```python
from build123d import *

# Parameters (mm, degrees)
SKETCH1_R           = 1.1303
SKETCH1_R_2         = 0.889
SKETCH1_W           = 5
SKETCH1_H           = 8.000000002
BOSS_EXTRUDE1_DEPTH = 6.35


with BuildPart() as part:
    # Sketch1 → Boss-Extrude1 (new body)
    with BuildSketch(Plane.XY):
        with BuildLine():
            Line((-16.134535362, 9.317270845), (-16.134535362, -47.832729155))
            Line((-16.134535362, -47.832729155), (-9.784535362, -47.832729155))
            Line((-9.784535362, -47.832729155), (-9.784535362, -41.482729155))
            Line((-9.784535362, -41.482729155), (-3.434535362, -41.482729155))
            Line((-3.434535362, -41.482729155), (-3.434535362, -47.832729155))
            Line((-3.434535362, -47.832729155), (15.615464638, -47.832729155))
            Line((15.615464638, -47.832729155), (15.615464638, -41.482729155))
            Line((15.615464638, -41.482729155), (21.965464638, -41.482729155))
            Line((21.965464638, -41.482729155), (21.965464638, 9.317270845))
            ThreePointArc((21.965464638, 9.317270845), (18.245720759, 18.297526966), (9.265464638, 22.017270845))
            Line((9.265464638, 22.017270845), (-16.134535362, 22.017270845))
            Line((-16.134535362, 22.017270845), (-16.134535362, 15.667270845))
            Line((-16.134535362, 15.667270845), (-9.784535362, 15.667270845))
            Line((-9.784535362, 15.667270845), (-9.784535362, 9.317270845))
            Line((-9.784535362, 9.317270845), (-16.134535362, 9.317270845))
        make_face()
        with Locations((-2.164535362, -35.132729155)):
            Circle(SKETCH1_R, mode=Mode.SUBTRACT)
        with Locations((-2.164535362, 1.867270845)):
            Circle(SKETCH1_R, mode=Mode.SUBTRACT)
        with Locations((12.440464638, -44.657729155)):
            Circle(SKETCH1_R_2, mode=Mode.SUBTRACT)
        with Locations((-12.959535362, -35.132729155)):
            Circle(SKETCH1_R_2, mode=Mode.SUBTRACT)
        with Locations((13.035464638, -16.63272908)):
            Rectangle(SKETCH1_W, SKETCH1_H, mode=Mode.SUBTRACT)
    extrude(amount=BOSS_EXTRUDE1_DEPTH)


solid = part.part
```
Can you work these out from the model? Positions are in its coordinate system, mm. A direction names the side the tool comes from. Round coordinates to 2 decimals unless told otherwise and drop trailing zeros. Order: outer loops, then holes, each group sorted by start corner. A loop starts at its lowest first (then second) coordinate and runs counter-clockwise, first axis right, second up.
(1) If we section it at A-A (y = -14): Please give me the cut outline in (x, z), plus the area to 3 significant figures.
Results are:
outline: (-16.13, 0) - (10.54, 0) - (10.54, 6.35) - (-16.13, 6.35) - close; (15.54, 0) - (21.97, 0) - (21.97, 6.35) - (15.54, 6.35) - close
area: 210 mm2
(2) If we section it at C-C (z = 2.25): Please give me the cut outline in (x, y), plus the area to 3 significant figures.
Results are:
outline: (-16.13, -47.83) - (-9.78, -47.83) - (-9.78, -41.48) - (-3.43, -41.48) - (-3.43, -47.83) - (15.62, -47.83) - (15.62, -41.48) - (21.97, -41.48) - (21.97, 9.32) arc R12.7 ccw to (9.27, 22.02) - (-16.13, 22.02) - (-16.13, 15.67) - (-9.78, 15.67) - (-9.78, 9.32) - (-16.13, 9.32) - close; hole circle Ø1.78 at (-12.96, -35.13); hole circle Ø2.26 at (-2.16, -35.13); hole circle Ø2.26 at (-2.16, 1.87); hole (10.54, -20.63) - (15.54, -20.63) - (15.54, -12.63) - (10.54, -12.63) - close; hole circle Ø1.78 at (12.44, -44.66)
area: 2,450 mm2
(3) On a 3-axis mill with a long thin cutter (end or side, diameter ignored), from which of +Z, -Z, +X, -X, +Y, -Y can I reach the whole of each face in a straight line? I mean faces 4 (the face through (-13, 15.667, 3)), 5 (the face through (19, -41.483, 3)), 6 (the face through (-16.135, -19, 3)), 7 (the face through (-7, -41.483, 3)), 8 (the face through (13, -12.633, 3)). Say none if no direction works.
Results are:
face 4: +Z, -Z, -X
face 5: +Z, -Z, +X, -Y
face 6: +Z, -Z, -X, +Y, -Y
face 7: +Z, -Z, -Y
face 8: +Z, -Z
(4) If we section it at D-D (x = 16.5): Please give me the cut outline in (y, z).
Results are:
outline: (-41.48, 0) - (19.76, 0) - (19.76, 6.35) - (-41.48, 6.35) - close
(5) If we section it at B-B (x = -2): Please give me the cut outline in (y, z), plus the area to 3 significant figures.
Results are:
outline: (-47.83, 0) - (-36.25, 0) - (-36.25, 6.35) - (-47.83, 6.35) - close; (-34.01, 0) - (0.75, 0) - (0.75, 6.35) - (-34.01, 6.35) - close; (2.99, 0) - (22.02, 0) - (22.02, 6.35) - (2.99, 6.35) - close
area: 415 mm2
(6) I'm going to push flat-ended pins straight in: pin 1 (2 mm diameter, centred on y = 11, z = 1, fed in from -X); pin 2 (3 mm diameter, centred on y = -44, z = 4, fed in from +X). Where does each tip first touch, or does it pass through?
Results are:
pin 1: stops at x = -9.78
pin 2: stops at x = 15.62
(7) We'd pull the mould along X, two halves only. Please class faces 1 (the face through (18.34, 18.2, 3.13)), 2 (the face through (13.26, -45, 3.13)), 3 (the face through (-13, -47.833, 3)): +X half, -X half, draft (parallel to the pull), parting line (faces both ways), or undercut.
Results are:
face 1: +X half
face 2: undercut
face 3: draft
(8) If I drill on L1, parallel to Y at x = -13, z = 6.25; L2, parallel to X at y = -42, z = 5.5; L3, parallel to Y at x = -11.5, z = 1.25, over which ranges is the centre line in solid material (lowest first)?
Results are:
L1: y = -47.83 to -36.02, -34.24 to 9.32, 15.67 to 22.02
L2: x = -16.13 to -9.78, -3.43 to 15.62
L3: y = -47.83 to 9.32, 15.67 to 22.02
